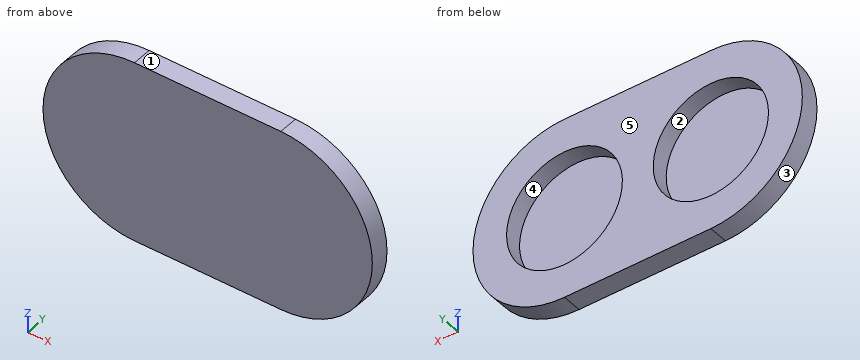
from build123d import *

# Parameters (mm, degrees)
SKETCH1_R           = 10
SKETCH1_R_2         = 10.05
BOSS_EXTRUDE1_DEPTH = 3.4
SKETCH1_2_R         = 10
SKETCH1_2_R_2       = 10.05
BOSS_EXTRUDE2_DEPTH = 0.4


with BuildPart() as part:
    # Sketch1 → Boss-Extrude1 (new body)
    with BuildSketch(Plane(origin=(0, 0, 0), x_dir=(1, 0, 0), z_dir=(0, 1, 0))):
        with BuildLine():
            Line((0, 15.875), (25.4, 15.875))
            ThreePointArc((25.4, 15.875), (41.275, 0), (25.4, -15.875))
            Line((25.4, -15.875), (0, -15.875))
            ThreePointArc((0, -15.875), (-15.875, 0), (0, 15.875))
        make_face()
        with Locations(Location((0, 0, 0), (0, 0, 270))):
            Circle(SKETCH1_R, mode=Mode.SUBTRACT)
        with Locations(Location((25.4, 0, 0), (0, 0, 270))):
            Circle(SKETCH1_R_2, mode=Mode.SUBTRACT)
    extrude(amount=BOSS_EXTRUDE1_DEPTH)

    # Sketch1_2 → Boss-Extrude2 (add)
    with BuildSketch(Plane(origin=(0, 0, 0), x_dir=(1, 0, 0), z_dir=(0, 1, 0))):
        with Locations(Location((0, 0, 0), (0, 0, 270))):
            Circle(SKETCH1_2_R)
        with Locations(Location((25.4, 0, 0), (0, 0, 270))):
            Circle(SKETCH1_2_R_2)
    extrude(amount=BOSS_EXTRUDE2_DEPTH)


solid = part.part
Input: part model. Units: mm. Frame: model coordinates. Face numbers are marked on the shaded views. A direction names the side the tool comes from. Give positions to 0.01 mm unless a question says otherwise; leave off trailing zeros. Order: outer loops, then holes, each group sorted by start corner. A loop starts at its lowest first (then second) coordinate and runs counter-clockwise, first axis right, second up. Notation, with made-up numbers: (-15.5, 51) - (28.5, 51) arc R18 ccw to (28.5, 62) - close; hole circle Ø9 at (38.5, -23). An arc over 180 degrees is marked (long way). Answer as a JSON object with one key per item and string values. Group by question number.
Q1. Cut plane C-C, the plane x = 5. Output: boundary loops of the cut face in (y, z) (3 decimals), then the cut area to 3 significant figures.
Q2. Mould query, pull axis X, two halves, no side actions, for the marked faces 3, 4 and 5. Classes: pulls with the +X half, pulls with the -X half, needs draft (parallel to the pull), parting line crosses it, or undercut.
Q3. Cut plane D-D, the plane z = -7. Output: boundary loops of the cut face in (x, y).
Q4. Line query: probe 1 along X at (y, z) = (2.1, 0) (3 decimals); probe 2 along X at (y, z) = (1.4, -2.5); probe 3 along Z at (x, y) = (6, 2.25) (3 decimals). Output: solid intervals per line, ascending.
Q5. First-contact query: pin 1 Ø10 at (x, z) = (2, -2.5) entering from +Y; pin 2 Ø2 at (y, z) = (1.5, -2.5) entering from -X. Flat tips, straight axial feed; report the tip coordinate or a pass-through.
Q6. Set-up query: the marked faces 1 and 2. Return all of +Z, -Z, +X, -X, +Y, -Y with unobstructed straight access to the full face (end or side cutting, diameter ignored); none if empty.
Q7. Cut plane B-B, the plane y = 2.2. Output: boundary loops of the cut face in (x, z) (3 decimals).
Q8. Cut plane A-A, the plane z = 0. Output: boundary loops of the cut face in (x, y) (3 decimals), then the cut area to 3 significant figures.
Results:
{
 "1": {"outline": "(0, -15.875) - (3.4, -15.875) - (3.4, -8.66) - (0.4, -8.66) - (0.4, 8.66) - (3.4, 8.66) - (3.4, 15.875) - (0, 15.875) - close", "area": "56.0 mm^2"},
 "2": {"face 3": "pulls with the -X half", "face 4": "undercut", "face 5": "needs draft"},
 "3": {"outline": "(-14.25, 0) - (39.65, 0) - (39.65, 3.4) - (32.61, 3.4) - (32.61, 0.4) - (18.19, 0.4) - (18.19, 3.4) - (7.14, 3.4) - (7.14, 0.4) - (-7.14, 0.4) - (-7.14, 3.4) - (-14.25, 3.4) - close"},
 "4": {"probe 1": "-15.875 to -10, 10 to 15.35, 35.45 to 41.275", "probe 2": "-15.68 to -9.68, 9.68 to 15.67, 35.13 to 41.08", "probe 3": "-15.875 to -8, 8 to 15.875"},
 "5": {"pin 1": "y = 0.4", "pin 2": "x = -15.8"},
 "6": {"face 1": "+Z, +X, -X, +Y, -Y", "face 2": "+Y"},
 "7": {"outline": "(0, -15.875) - (25.4, -15.875) arc R15.875 ccw to (25.4, 15.875) - (0, 15.875) arc R15.875 ccw to start; hole circle Ø20 at (0, 0); hole circle Ø20.1 at (25.4, 0)"},
 "8": {"outline": "(-15.875, 0) - (41.275, 0) - (41.275, 3.4) - (35.45, 3.4) - (35.45, 0.4) - (15.35, 0.4) - (15.35, 3.4) - (10, 3.4) - (10, 0.4) - (-10, 0.4) - (-10, 3.4) - (-15.875, 3.4) - close", "area": "74.0 mm^2"}
}
